Drawing for the job (mm, zero at the part's lowest x, y, z). Round coordinates to 2 decimals unless told otherwise and drop trailing zeros. Write each loop counter-clockwise with the first axis right and the second up, starting at its lowest first coordinate (ties: lowest second). Pieces come first, ordered by that corner, then holes. Notation, with made-up numbers: M -21.5,54 L 7.5,54 A28 ccw 7.5,88 Z; hole C -2.75,37 d8. An arc over 180 degrees is marked long. Use a Markdown table: item, result. Add a question column.
1) Slice it at A-A on x = 2. Write the cut outline in (y, z).
2) Two-plate mould, pull along Y, no slides. Class the marked faces 1, 2 and 3: released by +Y, released by -Y, zero draft, split by the parting line, or undercut.
3) Drop flat-ended pins along their axis: P1, Ø1.5, axis at x = 14, z = 22.5, coming from the -Y side; P2, Ø6, axis at x = 2.5, z = 17, coming from the -Y side; P3, Ø1.5, axis at y = 3.5, z = 15, coming from the -X side (1 decimal). Give the stop position or say it passes through.
4) Slice it at C-C on y = 17. Write the cut outline in (x, z), plus the area to 3 significant figures.
5) Slice it at D-D on x = 20.25. Write the cut outline in (y, z).
6) Slice it at B-B on z = 22.75. Write the cut outline in (x, y) (1 decimal).
7) Wall check: probe 1 along Y at (x, z) = (19.5, 23.75) (1 decimal); probe 2 along Y at (x, z) = (12.25, 1.5); probe 3 along Y at (x, z) = (22, 7.75) (1 decimal). Give the ranges that are in metal, low to high.
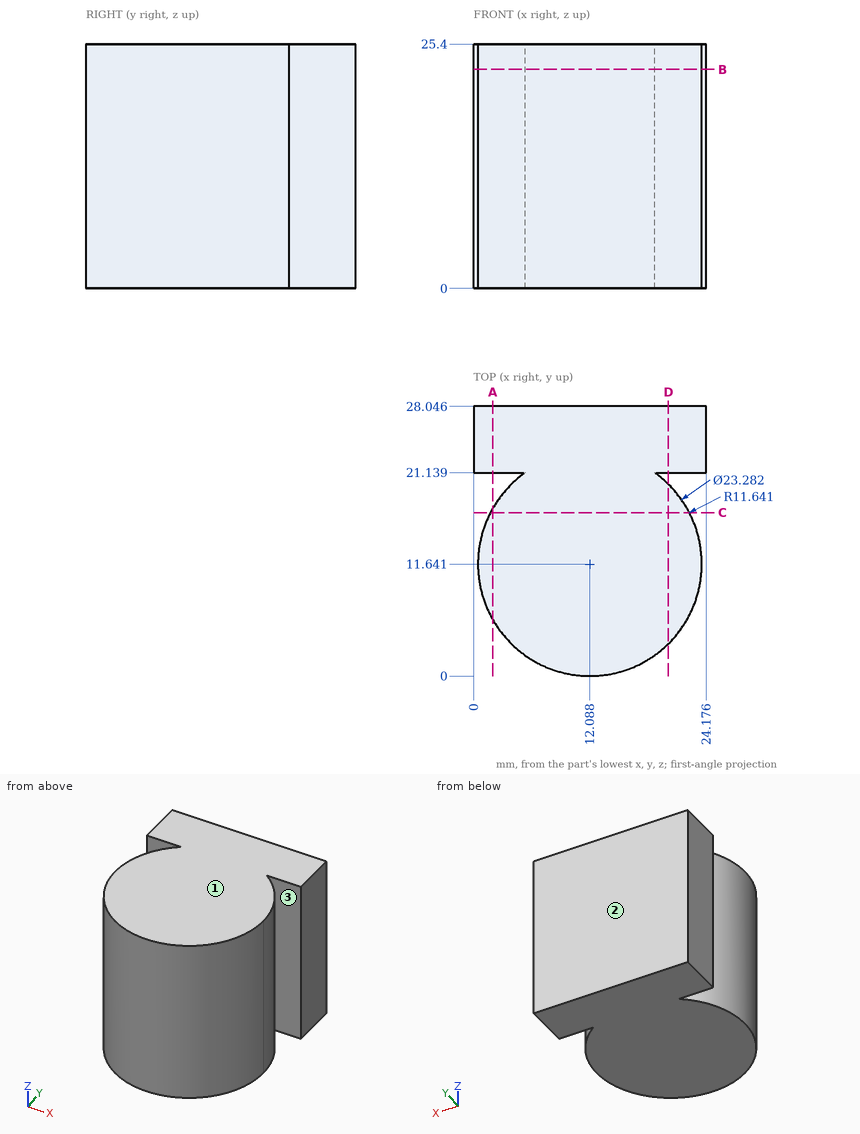
Entries:
| question | item | result |
|---|---|---|
| 1 | outline | M 5.83,0 L 17.45,0 L 17.45,25.4 L 5.83,25.4 Z; M 21.14,0 L 28.05,0 L 28.05,25.4 L 21.14,25.4 Z |
| 2 | face 1 | zero draft |
| 2 | face 2 | released by +Y |
| 2 | face 3 | undercut |
| 3 | P1 | stops at y = 0.06 |
| 3 | P2 | stops at y = 2.04 |
| 3 | P3 | stops at x = 3.1 |
| 4 | outline | M 1.75,0 L 22.42,0 L 22.42,25.4 L 1.75,25.4 Z |
| 4 | area | 525 mm^2 |
| 5 | outline | M 3.34,0 L 19.94,0 L 19.94,25.4 L 3.34,25.4 Z; M 21.14,0 L 28.05,0 L 28.05,25.4 L 21.14,25.4 Z |
| 6 | outline | M 0,21.1 L 5.4,21.1 A11.6 ccw long 18.8,21.1 L 24.2,21.1 L 24.2,28 L 0,28 Z |
| 7 | probe 1 | y = 2.7 to 20.6, 21.1 to 28 |
| 7 | probe 2 | y = 0 to 28.05 |
| 7 | probe 3 | y = 5.5 to 17.7, 21.1 to 28 |
